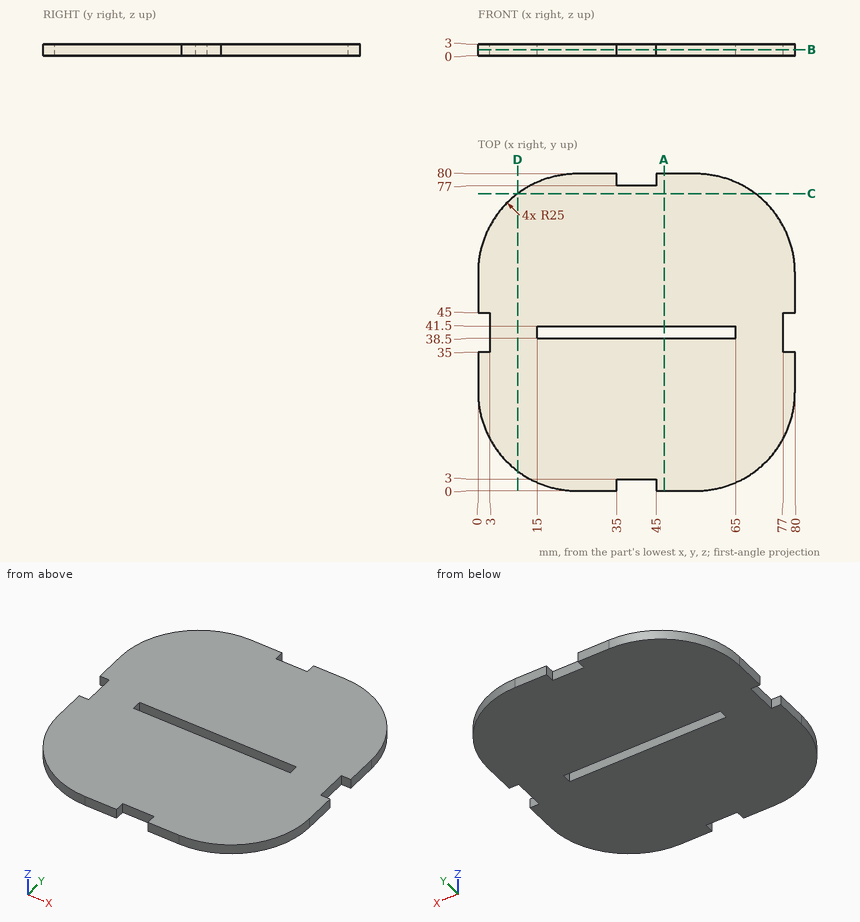
Job drawing, mm, ordinate dimensions from the low corner. One solid piece. Give positions to 0.01 mm unless a question says otherwise; leave off trailing zeros. Loops run counter-clockwise (first coordinate to the right, second up) from the corner with the lowest first, then second, coordinate; pieces in that order, holes last. Notation, with made-up numbers: (17.5, -29) -> (61.5, -29) arc R10 cw to (61.5, -19) -> close; hole circle Ø9 at (-8, -9). An arc over 180 degrees is marked (long way). Write each question's results on one line, items separated by ' | '.
(1) Cut at A-A on x = 47. List the corners of the cut face in (y, z), and give its area (3 significant figures).
Geometry results:
outline: (0, 0) -> (38.5, 0) -> (38.5, 3) -> (0, 3) -> close; (41.5, 0) -> (80, 0) -> (80, 3) -> (41.5, 3) -> close | area: 231 mm²
(2) Cut at C-C on y = 75. List the corners of the cut face in (x, z), and give its area (3 significant figures).
Geometry results:
outline: (10, 0) -> (70, 0) -> (70, 3) -> (10, 3) -> close | area: 180 mm²
(3) Cut at B-B on z = 1.6. List the corners of the cut face in (x, y).
Geometry results:
outline: (0, 25) arc R25 ccw to (25, 0) -> (35, 0) -> (35, 3) -> (45, 3) -> (45, 0) -> (55, 0) arc R25 ccw to (80, 25) -> (80, 35) -> (77, 35) -> (77, 45) -> (80, 45) -> (80, 55) arc R25 ccw to (55, 80) -> (45, 80) -> (45, 77) -> (35, 77) -> (35, 80) -> (25, 80) arc R25 ccw to (0, 55) -> (0, 45) -> (3, 45) -> (3, 35) -> (0, 35) -> close; hole (15, 38.5) -> (65, 38.5) -> (65, 41.5) -> (15, 41.5) -> close
(4) Cut at D-D on x = 10. List the corners of the cut face in (y, z).
Geometry results:
outline: (5, 0) -> (75, 0) -> (75, 3) -> (5, 3) -> close
(5) Flat gauge pins, fed straight in: pin 1 Ø1.5 at (x, z) = (2, 1) entering from -Y; pin 2 Ø1 at (x, z) = (40, 1) entering from -Y; pin 3 Ø1.5 at (y, z) = (39, 1.5) entering from -X. Where does each tip first touch, or does it go through?
Geometry results:
pin 1: stops at y = 13.6 | pin 2: stops at y = 3 | pin 3: stops at x = 3
(6) Probe line 1 along Y through (x, z) = (35.5, 1.75); line 2 along Y through (x, z) = (47.5, 2.15); line 3 along X through (y, z) = (35.5, 2.2). List the from-to ranges inside material, lowest first.
Geometry results:
line 1: y = 3 to 38.5, 41.5 to 77 | line 2: y = 0 to 38.5, 41.5 to 80 | line 3: x = 3 to 77
